Source: CAD feature listing. Evaluate the final solid. Frame: model axes, mm. A direction names the side the tool comes from. Give positions to 0.01 mm unless a question says otherwise; leave off trailing zeros. Order: outer loops, then holes, each group sorted by start corner. A loop starts at its lowest first (then second) coordinate and runs counter-clockwise, first axis right, second up. Notation, with made-up numbers: (87, -13.75) -> (136, -13.75) arc R20 ccw to (136, 14.25) -> close; hole circle Ø9 at (70.25, -16.5). An arc over 180 degrees is marked (long way). Answer in a Markdown table with one row per item.
```python
from build123d import *

# Parameters (mm, degrees)
ESQUISSE3_R             = 2.35
BOSS_EXTRU_2_DEPTH      = 70.2
CHANFREIN1_SIZE         = 5
ESQUISSE6_R             = 3.2
ESQUISSE6_R_2           = 2.35
ENL_V_MAT_EXTRU_1_DEPTH = 7
ENL_V_START             = -7
ESQUISSE7_R             = 3.2
ESQUISSE7_R_2           = 2.35
ENL_V_MAT_EXTRU_2_DEPTH = 7


with BuildPart() as part:
    # Esquisse3 → Boss.-Extru.2 (new, symmetric)
    with BuildSketch(Plane(origin=(0, 0, 0), x_dir=(0, 0, -1), z_dir=(1, 0, 0))):
        Polygon((-4.5, -10.5), (-4.5, 4.5), (10.5, 4.5), (10.5, -4.5), (4.5, -4.5), (4.5, -10.5), align=None)
        with Locations((1.5, -1.5)):
            Circle(ESQUISSE3_R, mode=Mode.SUBTRACT)
    extrude(amount=BOSS_EXTRU_2_DEPTH, both=True)

    # Chanfrein1
    chanfrein1_edges = [part.edges().sort_by_distance(p)[0] for p in [
        (0, 4.5, 4.5),
    ]]
    chamfer(chanfrein1_edges, length=CHANFREIN1_SIZE)

    # Esquisse6 → Enlèv. mat.-Extru.1 (cut)
    with BuildSketch(Plane.ZY.offset(70.2)):
        with Locations((-1.5, -1.5)):
            Circle(ESQUISSE6_R)
        with Locations((-1.5, -1.5)):
            Circle(ESQUISSE6_R_2, mode=Mode.SUBTRACT)
    extrude(amount=-ENL_V_MAT_EXTRU_1_DEPTH, mode=Mode.SUBTRACT)

    # Esquisse7 → Enlèv. mat.-Extru.2 (cut)
    with BuildSketch(Plane(origin=(70.2, 0, 0), x_dir=(0, 0, -1), z_dir=(1, 0, 0)).offset(ENL_V_START)):
        with Locations(Location((1.5, -1.5, 0), (0, 0, 180))):
            Circle(ESQUISSE7_R)
        with Locations(Location((1.5, -1.5, 0), (0, 0, 180))):
            Circle(ESQUISSE7_R_2, mode=Mode.SUBTRACT)
    extrude(amount=ENL_V_MAT_EXTRU_2_DEPTH, mode=Mode.SUBTRACT)


solid = part.part
```
(1) Section query C-C (y = -7.25). Return the cut outline in (x, z).
A:
| item | result |
|---|---|
| outline | (-70.2, -4.5) -> (70.2, -4.5) -> (70.2, 4.5) -> (-70.2, 4.5) -> close |
(2) Access query for faces 4 (the flat face through (1, 2, 2)), 5 (the flat face through (1, -4.5, -8)), 6 (the flat face through (-63.2, 1, -2)), 7 (the flat face through (70.2, -3, -5)), 8 (the cylindrical face through (66.651, -0.274, 1.456)). Directions: +Z, -Z, +X, -X, +Y, -Y. A direction counts if a zero-diameter tool reaches every point of the face in a straight line with its end or side. Return the directions, or none.
A:
| item | result |
|---|---|
| face 4 | +Z, +X, -X, +Y |
| face 5 | -Z, +X, -X, -Y |
| face 6 | -X |
| face 7 | +Z, -Z, +X, +Y, -Y |
| face 8 | +X |
(3) Section query B-B (z = -2.5). Return the cut outline in (x, y), plus the area to 3 significant figures.
A:
| item | result |
|---|---|
| outline | (-70.2, -10.5) -> (70.2, -10.5) -> (70.2, -4.54) -> (63.2, -4.54) -> (63.2, -3.63) -> (-63.2, -3.63) -> (-63.2, -4.54) -> (-70.2, -4.54) -> close; (-70.2, 1.54) -> (-63.2, 1.54) -> (-63.2, 0.63) -> (63.2, 0.63) -> (63.2, 1.54) -> (70.2, 1.54) -> (70.2, 4.5) -> (-70.2, 4.5) -> close |
| area | 1,480 mm^2 |
(4) First-contact query: pin 1 Ø6 at (y, z) = (-1.5, -1.5) entering from +X; pin 2 Ø3 at (y, z) = (-1.5, -1) entering from -X (1 decimal); pin 3 Ø1 at (x, z) = (38.5, -5.5) entering from -Y; pin 4 Ø6.5 at (x, y) = (26.5, -9) entering from -Z. Flat tips, straight axial feed; report the tip coordinate or a pass-through.
A:
| item | result |
|---|---|
| pin 1 | stops at x = 63.2 |
| pin 2 | passes through |
| pin 3 | stops at y = -4.5 |
| pin 4 | stops at z = -4.5 |
(5) Ray query, probe 1 along Y at (x, z) = (9.5, -1.5); probe 2 along Y at (x, z) = (37, -7.25). Return the intervals inside material, ascending.
A:
| item | result |
|---|---|
| probe 1 | y = -10.5 to -3.85, 0.85 to 4.5 |
| probe 2 | y = -4.5 to 4.5 |
(6) Section query A-A (x = 41.5). Return the cut outline in (y, z), plus the area to 3 significant figures.
A:
| item | result |
|---|---|
| outline | (-10.5, -4.5) -> (-4.5, -4.5) -> (-4.5, -10.5) -> (4.5, -10.5) -> (4.5, -0.5) -> (-0.5, 4.5) -> (-10.5, 4.5) -> close; hole circle Ø4.7 at (-1.5, -1.5) |
| area | 159 mm^2 |
(7) Pull-direction query (Z, two-part tool) for faces 1 (the cylindrical face through (-0.885, -1.397, 0.848)), 2 (the flat face through (1, 4.5, -5)), 3 (the flat face through (1, -7, -4.5)); classes: +Z half, -Z half, draft (parallel to the pull), parting line (faces both ways), or undercut.
A:
| item | result |
|---|---|
| face 1 | undercut |
| face 2 | draft |
| face 3 | -Z half |
